Autodesk Inventor part; units mm, degrees
ref_plane "YZ Plane" through (0, 0, 0) normal (1, 0, 0) x (0, 1, 0)
ref_plane "XZ Plane" through (0, 0, 0) normal (0, 1, 0) x (-1, 0, 0)
ref_plane "XY Plane" through (0, 0, 0) normal (0, 0, 1) x (1, 0, 0)
sketch "Sketch1" plane through (0, 0, 0) normal (0, 0, 1) x (1, 0, 0)
  line L0 (-15, -9.5) -> (15, -9.5)
  line L1 (15, -9.5) -> (15, 9.5)
  line L2 (15, 9.5) -> (-15, 9.5)
  line L3 (-15, 9.5) -> (-15, -9.5)
  point P0 (0, 0)
  point P1 (0, 9.5)
  point P2 (15, 0)
  dimension "d0" = 30
  dimension "d1" = 19
extrude "Extrusion1" add sketch "Sketch1" along normal blind 3
sketch "Sketch2" plane through (0, 0, 0) normal (0, 0, -1) x (-1, 0, 0)
  line L0 (-12.7, -5.93) -> (12.7, -5.93)
  line L1 (12.7, -5.93) -> (12.7, -8.47)
  line L2 (12.7, -8.47) -> (-12.7, -8.47)
  line L3 (-12.7, -8.47) -> (-12.7, -5.93)
  line L4 (15, -9.5) -> (-15, -9.5)
  circle A0 centre (-11.46, -7.2) radius 0.5
  circle A1 centre (-8.92, -7.2) radius 0.5
  circle A2 centre (-6.38, -7.2) radius 0.5
  circle A3 centre (-3.84, -7.2) radius 0.5
  circle A4 centre (-1.3, -7.2) radius 0.5
  circle A5 centre (1.24, -7.2) radius 0.5
  circle A6 centre (3.78, -7.2) radius 0.5
  circle A7 centre (6.32, -7.2) radius 0.5
  circle A8 centre (8.86, -7.2) radius 0.5
  circle A9 centre (11.4, -7.2) radius 0.5
  line L5 (15, 9.5) -> (15, -9.5)
  point P0 (0, 0)
  point P1 (-12.7, -7.2)
  point P2 (0, -5.93)
  point P3 (12.7, -7.2)
  dimension "d4" = 2.3
  dimension "d5" = 2.54
  dimension "d6" = 25.4
  dimension "d7" = 3.6
  dimension "d8" = 2.54
  dimension "d9" = 2.54
  dimension "d10" = 2.54
  dimension "d11" = 2.54
  dimension "d12" = 2.54
  dimension "d13" = 2.54
  dimension "d14" = 2.54
  dimension "d15" = 2.54
  dimension "d16" = 2.54
  dimension "d17" = 1
extrude "Extrusion2" add sketch "Sketch2" along normal blind 2.54
equation "\"d9\" = d8"
equation "\"d10\" = d8"
equation "\"d11\" = d8"
equation "\"d12\" = d8"
equation "\"d13\" = d8"
equation "\"d14\" = d8"
equation "\"d15\" = d8"
equation "\"d16\" = d8"
properties part number "IMU"
Source: CAD feature listing. Evaluate the final solid. Frame: model axes, mm. A direction names the side the tool comes from. Give positions to 0.01 mm unless a question says otherwise; leave off trailing zeros. Order: outer loops, then holes, each group sorted by start corner. A loop starts at its lowest first (then second) coordinate and runs counter-clockwise, first axis right, second up.
(1) Section query A-A (x = -7.25). Return the cut outline in (y, z), plus the area to 3 significant figures.
(2) Contact query for flat-ended pins moving along their axis: P1, Ø1.3, axis at x = 3.5, z = -1, coming from the -Y side; P2, Ø3, axis at x = 12, y = 4.5, coming from the -Z side. Output: stop coordinate, or through.
(3) Section query B-B (y = 0.25). Return the cut outline in (x, z).
(4) Access query for faces 1 (the face through (15, 0, 1)), 2 (the face through (0, -5.93, -1)), 3 (the face through (3.57, -7.62, -1.25)). Directions: +Z, -Z, +X, -X, +Y, -Y. A direction counts if a zero-diameter tool reaches every point of the face in a straight line with its end or side. Return the directions, or none.
(5) Material intervals for line 1 along Y through (x, z) = (-8.86, -0.6); line 2 along Y through (x, z) = (10, -0.4); line 3 along Z through (x, y) = (1, -2), sorted ascending.
(6) Pull-direction query (X, two-part tool) for faces 4 (the face through (9, -7, 0)), 5 (the face through (0, -7, -2.54)), 6 (the face through (-12.7, -7, -1)), 7 (the face through (12.7, -7, -1)); classes: +X half, -X half, draft (parallel to the pull), parting line (faces both ways), or undercut.
Outcome:
1. outline: (-9.5, 0) - (-8.47, 0) - (-8.47, -2.54) - (-5.93, -2.54) - (-5.93, 0) - (9.5, 0) - (9.5, 3) - (-9.5, 3) - close
1. area: 63.5 mm2
2. P1: stops at y = -8.47
2. P2: stops at z = 0
3. outline: (-15, 0) - (15, 0) - (15, 3) - (-15, 3) - close
4. face 1: +Z, -Z, +X, +Y, -Y
4. face 2: -Z, +X, -X, +Y
4. face 3: -Z
5. line 1: y = -8.47 to -7.7, -6.7 to -5.93
5. line 2: y = -8.47 to -5.93
5. line 3: z = 0 to 3
6. face 4: undercut
6. face 5: draft
6. face 6: -X half
6. face 7: +X half
